from build123d import *

# Parameters (mm, degrees)
SKETCH_1_R               = 11
EXTRUDE_1_DEPTH          = 8
FILLET_1_R               = 100
FILLET_3_R               = 100
EXTRUDE_2_DEPTH          = 10
FILLET_2_R               = 10
CHAMFER_1_SIZE           = 5
SKETCH_4_R               = 13
CUT_EXTRUDE_1_DEPTH      = 0.7
SKETCH_5_R               = 2.75
CUT_EXTRUDE_2_DEPTH      = 514.540365546
SKETCH_6_R               = 6
CUT_EXTRUDE_3_DEPTH      = 4
CUT_EXTRUDE_4_DEPTH      = 514.758413114
CUT_EXTRUDE_4_DEPTH_BACK = 514.758413114
SKETCH_7_R               = 4.3


with BuildPart() as part:
    # 草图1 → 凸台-拉伸1 (new body)
    with BuildSketch(Plane.XY):
        Polygon((0, 280), (861.751390409, 0), (0, 0), (-100, 0), (-961.751390409, 0), (-100, 280), align=None)
        with Locations((200, 100)):
            Circle(SKETCH_1_R, mode=Mode.SUBTRACT)
        with Locations(Location((-300, 100, 0), (0, 0, 180))):
            Circle(SKETCH_1_R, mode=Mode.SUBTRACT)
    extrude(amount=EXTRUDE_1_DEPTH)

    # 圆角1
    fillet_1_edges = [part.edges().sort_by_distance(p)[0] for p in [
        (861.751390409, 0, 4),
    ]]
    fillet(fillet_1_edges, radius=FILLET_1_R)

    # 圆角3
    fillet_3_edges = [part.edges().sort_by_distance(p)[0] for p in [
        (-961.751390409, 0, 4),
    ]]
    fillet(fillet_3_edges, radius=FILLET_3_R)

    # 草图2 → 凸台-拉伸2 (add)
    with BuildSketch(Plane.XY):
        with BuildLine():
            Line((0, 280), (-100, 280))
            Line((-100, 280), (-361.277938379, 195.10565163))
            ThreePointArc((-361.277938379, 195.10565163), (-429.145073001, 84.356553496), (-330.376238942, 0))
            Line((-330.376238942, 0), (230.376238942, 0))
            ThreePointArc((230.376238942, 0), (329.145073001, 84.356553496), (261.277938379, 195.10565163))
            Line((261.277938379, 195.10565163), (0, 280))
        make_face()
        Polygon((10, 266.236180795), (122.241374643, 229.766747442), (10, 35.358983849), align=None, mode=Mode.SUBTRACT)
        with BuildLine():
            Line((230.376238942, 10), (30, 10))
            Line((30, 10), (151.410485182, 220.289128906))
            Line((151.410485182, 220.289128906), (258.187768435, 185.595086467))
            ThreePointArc((258.187768435, 185.595086467), (319.268189595, 85.920898146), (230.376238942, 10))
        make_face(mode=Mode.SUBTRACT)
        Polygon((-110, 266.236180795), (-110, 35.358983849), (-222.241374643, 229.766747442), align=None, mode=Mode.SUBTRACT)
        with BuildLine():
            Line((-358.187768435, 185.595086467), (-251.410485182, 220.289128906))
            Line((-251.410485182, 220.289128906), (-130, 10))
            Line((-130, 10), (-330.376238942, 10))
            ThreePointArc((-330.376238942, 10), (-419.268189595, 85.920898146), (-358.187768435, 185.595086467))
        make_face(mode=Mode.SUBTRACT)
    extrude(amount=-EXTRUDE_2_DEPTH)

    # 圆角2
    fillet_2_edges = [part.edges().sort_by_distance(p)[0] for p in [
        (-110, 35.358983849, -5),
        (-110, 266.236180795, -5),
        (-130, 10, -5),
        (10, 266.236180795, -5),
        (10, 35.358983849, -5),
        (151.410485182, 220.289128906, -5),
        (30, 10, -5),
        (-251.410485182, 220.289128906, -5),
        (122.241374643, 229.766747442, -5),
        (-222.241374643, 229.766747442, -5),
    ]]
    fillet(fillet_2_edges, radius=FILLET_2_R)

    # 倒角1
    chamfer_1_edges = [part.edges().sort_by_distance(p)[0] for p in [
        (-230.63896919, 237.552825815, 8),
        (130.63896919, 237.552825815, 8),
        (329.145073001, 84.356553496, 8),
        (-50, 0, 8),
        (-429.145073001, 84.356553496, 8),
        (-230.63896919, 237.552825815, -10),
        (130.63896919, 237.552825815, -10),
        (329.145073001, 84.356553496, -10),
        (-50, 0, -10),
        (-429.145073001, 84.356553496, -10),
    ]]
    chamfer(chamfer_1_edges, length=CHAMFER_1_SIZE)

    # 草图4 → 切除-拉伸1 (cut)
    with BuildSketch(Plane(origin=(0, 0, 0), x_dir=(-1, 0, 0), z_dir=(0, 0, -1))):
        with Locations((-200, 100)):
            Circle(SKETCH_4_R)
        with Locations((300, 100)):
            Circle(SKETCH_4_R)
    extrude(amount=-CUT_EXTRUDE_1_DEPTH, mode=Mode.SUBTRACT)

    # 草图5 → 切除-拉伸2 (cut, through all)
    with BuildSketch(Plane(origin=(0, 0, 0), x_dir=(-1, 0, 0), z_dir=(0, 0, -1))):
        with Locations((-200, 130)):
            Circle(SKETCH_5_R)
        with Locations((-200, 70)):
            Circle(SKETCH_5_R)
        with Locations((300, 130)):
            Circle(SKETCH_5_R)
        with Locations((300, 70)):
            Circle(SKETCH_5_R)
    extrude(amount=-CUT_EXTRUDE_2_DEPTH, mode=Mode.SUBTRACT)

    # 草图6 → 切除-拉伸3 (cut)
    with BuildSketch(Plane.XY.offset(8)):
        with Locations((200, 130)):
            Circle(SKETCH_6_R)
        with Locations((200, 70)):
            Circle(SKETCH_6_R)
        with Locations((-300, 130)):
            Circle(SKETCH_6_R)
        with Locations((-300, 70)):
            Circle(SKETCH_6_R)
    extrude(amount=-CUT_EXTRUDE_3_DEPTH, mode=Mode.SUBTRACT)

    # 草图7 → 切除-拉伸4 (cut, two sides: drawn at the far end of the back side and taken through both)
    with BuildSketch(Plane.XY.offset(8).offset(-CUT_EXTRUDE_4_DEPTH_BACK)):
        with Locations((64, 217)):
            Circle(SKETCH_7_R)
        with Locations((24, 217)):
            Circle(SKETCH_7_R)
        with Locations((64, 177)):
            Circle(SKETCH_7_R)
        with Locations((24, 177)):
            Circle(SKETCH_7_R)
        with Locations((64, 89)):
            Circle(SKETCH_7_R)
        with Locations((24, 89)):
            Circle(SKETCH_7_R)
        with Locations((64, 49)):
            Circle(SKETCH_7_R)
        with Locations((24, 49)):
            Circle(SKETCH_7_R)
        with Locations(Location((-124, 49, 0), (0, 0, 180))):
            Circle(SKETCH_7_R)
        with Locations(Location((-164, 49, 0), (0, 0, 180))):
            Circle(SKETCH_7_R)
        with Locations(Location((-124, 89, 0), (0, 0, 180))):
            Circle(SKETCH_7_R)
        with Locations(Location((-164, 89, 0), (0, 0, 180))):
            Circle(SKETCH_7_R)
        with Locations(Location((-124, 177, 0), (0, 0, 180))):
            Circle(SKETCH_7_R)
        with Locations(Location((-164, 177, 0), (0, 0, 180))):
            Circle(SKETCH_7_R)
        with Locations(Location((-124, 217, 0), (0, 0, 180))):
            Circle(SKETCH_7_R)
        with Locations(Location((-164, 217, 0), (0, 0, 180))):
            Circle(SKETCH_7_R)
    extrude(amount=CUT_EXTRUDE_4_DEPTH + CUT_EXTRUDE_4_DEPTH_BACK, mode=Mode.SUBTRACT)


solid = part.part
Build history of the part. All positions in model axes, mm. A direction names the side the tool comes from. Coordinates: 2 decimals unless noted, no trailing zeros. Put each result on its own line as item: value.
1. Drop flat-ended pins along their axis: P1, Ø14, axis at x = -124, y = 177, coming from the -Z side; P2, Ø5, axis at x = -229, z = -5.5, coming from the +Y side; P3, Ø11, axis at x = 200, y = 130, coming from the +Z side; P4, Ø14, axis at x = -164, y = 89, coming from the +Z side. Give the stop position or say it passes through.
Answer sheet:
P1: stops at z = 0
P2: stops at y = 238.88
P3: stops at z = 4
P4: stops at z = 8
2. Tool access for faces 4 (the face through (53, 186, 0)), 5 (the face through (-224.469, 236.892, 5.535)): list every direction of +Z, -Z, +X, -X, +Y, -Y with a clear straight run to the whole face (end or side of a thin tool).
Answer sheet:
face 4: -Z
face 5: +Z, -X, +Y
3. Probe line 1 along Y through (x, z) = (24, 4.25); line 2 along X through (y, z) = (130, 1.95); line 3 along Y through (x, z) = (-300, 5.2). List the from-to ranges inside material, lowest first. Write a range as [from, to].
Answer sheet:
line 1: y = [1.25, 44.7], [53.3, 84.7], [93.3, 172.7], [181.3, 212.7], [221.3, 270.89]
line 2: x = [-425.77, -302.75], [-297.25, 197.25], [202.75, 325.77]
line 3: y = [2.2, 64], [76, 89], [111, 124], [136, 212.7]
4. Saw through at A-A (y = 100). Give the number of separate pieces and of enclosed holes in the cut face, and give its area (3 significant figures).
Answer sheet:
separate pieces: 3
enclosed holes: 0
area: 7,770 mm^2
5. Pull direction X, two halves, no side cores. Call faces 1 (the face through (-424.13, 83.24, 7.76)), 2 (the face through (-151, 186, 0)), 3 (the face through (120.61, 238.15, 5.53)): pulls with the +X half, pulls with the -X half, needs draft (parallel to the pull), parting line crosses it, or undercut.
Answer sheet:
face 1: pulls with the -X half
face 2: undercut
face 3: pulls with the +X half
